The drawing under review shows one solid part. Ordinate dimensions are in mm from its lowest x, y, z. Round coordinates to 2 decimals unless told otherwise and drop trailing zeros. Loops run counter-clockwise (first coordinate to the right, second up) from the corner with the lowest first, then second, coordinate; pieces in that order, holes last. Notation, with made-up numbers: (61.5, -2.5) - (116.5, -2.5) arc R30 cw to (116.5, 27.5) - close; hole circle Ø4 at (84, 87.5). An arc over 180 degrees is marked (long way). Answer as CSV lines item,"result".
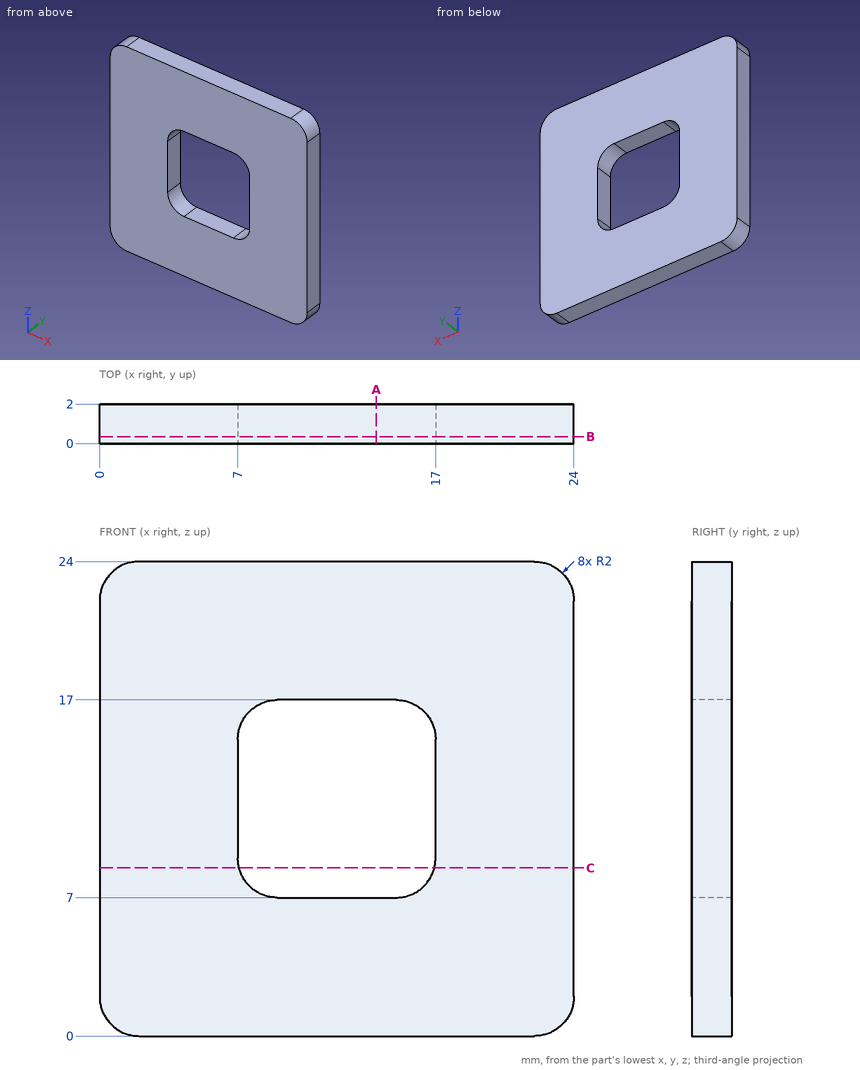
1. Take a section at A-A (x = 14). State the section outline as (y, z) points.
Numbers:
outline,"(0, 0) - (2, 0) - (2, 7) - (0, 7) - close; (0, 17) - (2, 17) - (2, 24) - (0, 24) - close"
2. Wall thickness on probe 1 along Z at (x, y) = (12.5, 1); probe 2 along X at (y, z) = (0.2, 16): over which ranges is each line inside the solid? List them lowest first.
Numbers:
probe 1,"z = 0 to 7, 17 to 24"
probe 2,"x = 0 to 7.27, 16.73 to 24"
3. Take a section at C-C (z = 8.5). State the section outline as (x, y) points.
Numbers:
outline,"(0, 0) - (7.06, 0) - (7.06, 2) - (0, 2) - close; (16.94, 0) - (24, 0) - (24, 2) - (16.94, 2) - close"
4. Take a section at B-B (y = 0.35). State the section outline as (x, z) points.
Numbers:
outline,"(0, 2) arc R2 ccw to (2, 0) - (22, 0) arc R2 ccw to (24, 2) - (24, 22) arc R2 ccw to (22, 24) - (2, 24) arc R2 ccw to (0, 22) - close; hole (7, 9) arc R2 ccw to (9, 7) - (15, 7) arc R2 ccw to (17, 9) - (17, 15) arc R2 ccw to (15, 17) - (9, 17) arc R2 ccw to (7, 15) - close"
